```python
from build123d import *

# Parameters (mm, degrees)
SKETCH1_R           = 90.805
BOSS_EXTRUDE1_DEPTH = 203.2
SKETCH2_W           = 80.01
SKETCH2_H           = 148.59
CUT_EXTRUDE1_DEPTH  = 203.2
SKETCH3_W           = 30
SKETCH3_H           = 85
CUT_EXTRUDE2_DEPTH  = 130
SKETCH4_R           = 15.24
CUT_EXTRUDE3_DEPTH  = 203.2
SKETCH5_R           = 15.24
CUT_EXTRUDE4_DEPTH  = 63.5


with BuildPart() as part:
    # Sketch1 → Boss-Extrude1 (new body)
    with BuildSketch(Plane(origin=(0, 0, 0), x_dir=(1, 0, 0), z_dir=(0, 1, 0))):
        with Locations(Location((0, 0, 0), (0, 0, 270))):
            Circle(SKETCH1_R)
    extrude(amount=BOSS_EXTRUDE1_DEPTH)

    # Sketch2 → Cut-Extrude1 (cut)
    with BuildSketch(Plane(origin=(0, 203.2, 0), x_dir=(1, 0, 0), z_dir=(0, 1, 0))):
        Rectangle(SKETCH2_W, SKETCH2_H)
    extrude(amount=-CUT_EXTRUDE1_DEPTH, mode=Mode.SUBTRACT)

    # Sketch3 → Cut-Extrude2 (cut)
    with BuildSketch(Plane(origin=(0, 203.2, 0), x_dir=(1, 0, 0), z_dir=(0, 1, 0))):
        with Locations((-59.45, 0)):
            Rectangle(SKETCH3_W, SKETCH3_H)
    extrude(amount=-CUT_EXTRUDE2_DEPTH, mode=Mode.SUBTRACT)

    # Sketch4 → Cut-Extrude3 (cut)
    with BuildSketch(Plane(origin=(0, 203.2, 0), x_dir=(1, 0, 0), z_dir=(0, 1, 0))):
        with Locations(Location((65.405, 0, 0), (0, 0, 270))):
            Circle(SKETCH4_R)
    extrude(amount=-CUT_EXTRUDE3_DEPTH, mode=Mode.SUBTRACT)

    # Sketch5 → Cut-Extrude4 (cut)
    with BuildSketch(Plane(origin=(0, 0, 0), x_dir=(-1, 0, 0), z_dir=(0, -1, 0))):
        with Locations((53.34, -3.393876065)):
            Circle(SKETCH5_R)
    extrude(amount=-CUT_EXTRUDE4_DEPTH, mode=Mode.SUBTRACT)


solid = part.part
```
Input: part model. Units: mm. Frame: model coordinates. A direction names the side the tool comes from. Coordinates: 2 decimals unless noted, no trailing zeros. Loops run counter-clockwise (first coordinate to the right, second up) from the corner with the lowest first, then second, coordinate; pieces in that order, holes last.
Q1. Section D-D, the plane z = -51.5. Return the cut outline in (x, y) (3 decimals), and give its area (3 significant figures).
Results are:
outline: (-74.788, 0) - (-40.005, 0) - (-40.005, 203.2) - (-74.788, 203.2) - close; (40.005, 0) - (74.788, 0) - (74.788, 203.2) - (40.005, 203.2) - close
area: 14,100 mm2
Q2. Section B-B, the plane z = 0. Return the cut outline in (x, y) (3 decimals), and give its area (3 significant figures).
Results are:
outline: (-90.805, 0) - (-68.197, 0) - (-68.197, 63.5) - (-40.005, 63.5) - (-40.005, 203.2) - (-44.45, 203.2) - (-44.45, 73.2) - (-74.45, 73.2) - (-74.45, 203.2) - (-90.805, 203.2) - close; (40.005, 0) - (50.165, 0) - (50.165, 203.2) - (40.005, 203.2) - close; (80.645, 0) - (90.805, 0) - (90.805, 203.2) - (80.645, 203.2) - close
area: 8,760 mm2
Q3. Set-up query: faces 1 (the flat face through (-1, 103, 74.295)), 2 (the flat face through (42, 203.2, -1)), 3 (the cylindrical face through (-68.57, 31.31, 3.96)), 4 (the flat face through (-60, 73.2, -1)). Return all of +Z, -Z, +X, -X, +Y, -Y with unobstructed straight access to the full face (end or side cutting, diameter ignored); none if empty.
Results are:
face 1: +Y, -Y
face 2: +Z, -Z, +X, -X, +Y
face 3: -Y
face 4: +Y
Q4. Contact query for flat-ended pins moving along their axis: pin 1 (15 mm diameter, centred on x = -58, y = 132.5, fed in from -Z); pin 2 (24 mm diameter, centred on x = -59.5, y = 128.5, fed in from +Z); pin 3 (1.5 mm diameter, centred on y = 159, z = 7, fed in from -X). Output: stop coordinate, or through.
Results are:
pin 1: stops at z = -75.47
pin 2: stops at z = 77.39
pin 3: stops at x = -90.59
Q5. Line query: line 1 along X through (y, z) = (41, 0) (3 decimals); line 2 along X through (y, z) = (106.5, 39) (3 decimals); line 3 along X through (y, z) = (121, 0) (3 decimals). Output: solid intervals per line, ascending.
Results are:
line 1: x = -90.805 to -68.197, 40.005 to 50.165, 80.645 to 90.805
line 2: x = -82.003 to -74.45, -44.45 to -40.005, 40.005 to 82.003
line 3: x = -90.805 to -74.45, -44.45 to -40.005, 40.005 to 50.165, 80.645 to 90.805
Q6. Section C-C, the plane y = 43. Return the cut outline in (x, z) (3 decimals).
Results are:
outline: circle Ø181.61 at (0, 0); hole (-40.005, -74.295) - (40.005, -74.295) - (40.005, 74.295) - (-40.005, 74.295) - (-40.005, 10.772) arc R15.24 ccw (long way) to (-40.005, -3.984) - close; hole circle Ø30.48 at (65.405, 0)
Q7. Section A-A, the plane x = 0. Return the cut outline in (y, z) (3 decimals).
Results are:
outline: (0, -90.805) - (203.2, -90.805) - (203.2, -74.295) - (0, -74.295) - close; (0, 74.295) - (203.2, 74.295) - (203.2, 90.805) - (0, 90.805) - close
Q8. Mould query, pull axis Z, two halves, no side actions, for faces 5 (the flat face through (42, 0, -1)), 6 (the flat face through (-54, 63.5, 3)), 7 (the cylindrical face through (90.032, 100.178, -11.821)). Classes: +Z half, -Z half, draft (parallel to the pull), parting line (faces both ways), or undercut.
Results are:
face 5: draft
face 6: undercut
face 7: parting line
